Autodesk Inventor part; units mm, degrees
ref_plane "YZ Plane" through (0, 0, 0) normal (1, 0, 0) x (0, 1, 0)
ref_plane "XZ Plane" through (0, 0, 0) normal (0, 1, 0) x (-1, 0, 0)
ref_plane "XY Plane" through (0, 0, 0) normal (0, 0, 1) x (1, 0, 0)
sketch "Boceto1" plane through (0, 0, 0) normal (0, 0, 1) x (1, 0, 0)
  line L0 (-103.5851, 10.8479) -> (31.8816, 10.8479) construction
  line L1 (31.8816, 10.8479) -> (31.8816, -10.8479) construction
  line L2 (31.8816, -10.8479) -> (-103.5851, -10.8479) construction
  line L3 (-103.5851, -10.8479) -> (-103.5851, 10.8479) construction
  line L4 (0, 0) -> (-71.5, 0)
  line L5 (0, 10.9) -> (0, 0)
  line L6 (-68.2708, 0) -> (0, 0)
  line L7 (0, 10.9) -> (-68.1013, 9.2541)
  line L8 (-71.5, 0) -> (-56.9274, 0) construction
  line L9 (-71.5, 0) -> (-71.5, 8.5)
  line L10 (-71.5, 0) -> (-68, 0)
  line L11 (-68, 0) -> (-68, 9.2565)
  arc A0 (-68, 9.2565) -> (-71.5, 8.5) centre (-67.8264, -0.0207) ccw
  line L12 (-68, 9.2565) -> (0, 10.9)
  line L13 (0, 0) -> (26.5, 0)
  line L14 (26.5, 0) -> (26.5, 7)
  line L15 (0, 0) -> (0, 9.9)
  line L16 (0, 0) -> (21, 0)
  line L17 (21, 0) -> (21, 9.5)
  line L18 (21, 9.5) -> (0, 9.9)
  line L19 (26.5, 0) -> (26.5, 8.5)
  arc A1 (26.5, 8.5) -> (21, 9.5) centre (21.692, -2.3188) ccw
  line L20 (26.5, 0) -> (29, 0)
  line L21 (29, 0) -> (29, 7)
  line L22 (29, 7) -> (26.5, 7)
  line L23 (29, 0) -> (29, 6.75)
  line L24 (29, 6.75) -> (31, 6.75)
  line L25 (31.8816, 6.75) -> (31.8816, 0)
  line L26 (31.8816, 0) -> (29, 0)
  line L27 (29, 0) -> (29, 6.75)
  line L28 (29, 6.75) -> (31, 6.75)
  line L29 (29, 0) -> (31, 0)
  ellipse E0 centre (31, 0) end of major axis (31, 6.75) minor radius 0.8816 (30.1184, 0) -> (31, 6.75) ccw
  ellipse E1 centre (31, 0) end of major axis (31, 6.75) minor radius 0.8816 (31, 6.75) -> (30.1184, 0) ccw
  line L30 (31, 6.75) -> (31.8816, 6.75)
  line L31 (-71.5, 0) -> (-71.5, 7.25)
  line L32 (-71.5, 0) -> (-67, 0)
  line L33 (-71.5, 0) -> (-76, 0)
  line L34 (-76, 0) -> (-76, 6.75)
  line L35 (-76, 6.75) -> (-71.5, 7.25)
  line L36 (-76, 0) -> (-77, 0)
  line L37 (-77, 0) -> (-77, 6.5)
  line L38 (-77, 6.5) -> (-76, 6.75)
  line L39 (-77, 0) -> (-80.5, 0)
  line L40 (-80.5, 0) -> (-80.5, 4.15)
  line L41 (-80.5, 4.15) -> (-77, 6.5)
  line L42 (-80.5, 0) -> (-87.5, 0)
  line L43 (-87.5, 0) -> (-87.5, 4.15)
  line L44 (-87.5, 4.15) -> (-80.5, 4.15)
  line L45 (-80.5, 4.15) -> (-80.5, 0)
  line L46 (-87.5, 0) -> (-95, 0)
  line L47 (-95, 0) -> (-95, 0)
  line L48 (-92.25, 2.75) -> (-87.5, 2.75)
  line L49 (-87.5, 2.75) -> (-87.5, 0)
  arc A2 (-92.25, 2.75) -> (-95, 0) centre (-92.25, 0) ccw
  point P0 (67.7333, -10.8479)
  point P1 (103.6012, -10.8479)
  point P2 (35.8517, 0)
  point P3 (7, 16)
  point P4 (-95, 2.75)
  dimension "d16" = 71.5
  dimension "d27" = 8.5
  dimension "d29" = 3.5
  dimension "d42" = 26.5
  dimension "d43" = 7
  dimension "d45" = 9.9
  dimension "d46" = 21
  dimension "d47" = 9.5
  dimension "d48" = 8.5
  dimension "d55" = 2.5
  dimension "d56" = 6.75
  dimension "d59" = 2
  dimension "d60" = 2
  dimension "d63" = 7.25
  dimension "d64" = 4.5
  dimension "d65" = 4.5
  dimension "d66" = 6.75
  dimension "d67" = 1
  dimension "d68" = 6.5
  dimension "d69" = 3.5
  dimension "d70" = 4.15
  dimension "d71" = 7
  dimension "d72" = 7.5
  dimension "d73" = 2.75
  dimension "d74" = 2.75
revolve "Revolución1" add sketch "Boceto1" angle 360 about axis through (0, 0, 0) along (-1, 0, 0) contours L4 L11 L7 L5 | L4 L9 A0 L7 L11
sketch "Boceto2" plane through (0, 0, 0) normal (1, 0, 0) x (0, 0, -1)
  arc A0 (1.1877, 9.8285) -> (-1.1877, 9.8285) centre (0, 0) ccw
  line L0 (0, 9.9) -> (0, 10.6)
  line L1 (0, 10.6) -> (0, 9.3)
  arc A1 (1.1877, 9.8285) -> (-1.1877, 9.8285) centre (0, 9.3) ccw
  arc A2 (-1.1877, 9.8285) -> (1.1877, 9.8285) centre (0, 0) ccw
  circle A3 centre (0, 9.3) radius 1.3
  point P0 (-1.1877, 9.8285)
  point P1 (1.1877, 9.8285)
  dimension "d38" = 19.8
  dimension "d39" = 0.7
  dimension "d40" = 1.3
revolve "Revolución2" add sketch "Boceto1" angle 360 about axis through (0, 0, 0) along (1, 0, 0) contours L5 L18 L17 L13 | L17 A1 L19 L14 L13
extrude "Extrusión1" add sketch "Boceto2" along normal blind 5 contours A3 A0 | A0 L0 A1 | A0 A1 L0
pattern_circular "Patrón circular1" count 12 over 360 about axis through (-10, 0, 0) along (1, 0, 0) of "Extrusión1"
revolve "Revolución3" add sketch "Boceto1" angle 360 about axis through (26.5, 0, 0) along (1, 0, 0) contours L14 L22 L21 L20 | L21 L24 E1 L26 | E1 E0 L26
revolve "Revolución4" add sketch "Boceto1" angle 360 about axis through (-80.5, 0, 0) along (-1, 0, 0) contours L33 L34 L35 L9 | L36 L37 L38 L34 | L39 L40 L41 L37 | L42 L43 L44 L40
revolve "Revolución5" add sketch "Boceto1" angle 360 about axis through (-87.5, 0, 0) along (-1, 0, 0) contours L46 A2 L48 L43
properties part number "marcador" material "Marcador Plastico"
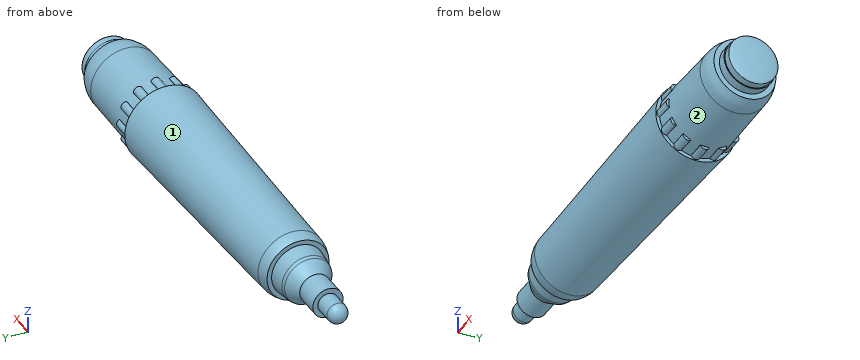
Design review of the part built by this model. Coordinates are the model's own, in mm. Face numbers are marked on the shaded views. A direction names the side the tool comes from. Give positions to 0.01 mm unless a question says otherwise; leave off trailing zeros. Write each loop counter-clockwise with the first axis right and the second up, starting at its lowest first coordinate (ties: lowest second). Pieces come first, ordered by that corner, then holes. Notation, with made-up numbers: M -3,57.25 L 47,57.25 A23 cw 47,84.25 Z; hole C 48.5,85.5 d4. An arc over 180 degrees is marked long. Answer as a JSON object with one key per item and string values. Group by question number.
1) We need section A-A (x = -84). Give the boundary of the cut face in (y, z), and give its area (3 significant figures).
2) Clearance check with flat-ended pins moving along their axes: pin 1 Ø6 at (y, z) = (4, -0.5) entering from +X; pin 2 Ø1 at (y, z) = (10.5, 0) entering from +X; pin 3 Ø10 at (x, z) = (-77, -6) entering from +Y. State where each tip first meets the part, or that it passes through.
3) For line 1 along Y through (x, z) = (-7, -5.75); line 2 along Y through (x, z) = (-62.5, -6.75); line 3 along X through (y, z) = (-6.75, 3), list the stretches that pass through material, from the lowest coordinate up.
4) Tool access review of the marked faces 1 and 2: name each direction out of +Z, -Z, +X, -X, +Y, -Y from which nothing blocks a thin tool from reaching the whole face with its end or side.
5) We need section B-B (x = 9). Give the boundary of the cut face in (y, z), and give its area (3 significant figures).
Answer key:
{
 "1": {"outline": "C 0,0 d8.3", "area": "54.1 mm²"},
 "2": {"pin 1": "stops at x = 31.87", "pin 2": "stops at x = 5", "pin 3": "stops at y = 6.72"},
 "3": {"line 1": "y = -9.06 to 9.06", "line 2": "y = -6.53 to 6.53", "line 3": "x = -71.5 to 26.5"},
 "4": {"face 1": "-X", "face 2": "+X"},
 "5": {"outline": "C 0,0 d19.46", "area": "297 mm²"}
}
